Build history of the part. All positions in model axes, mm. A direction names the side the tool comes from. Coordinates: 2 decimals unless noted, no trailing zeros. Loops run counter-clockwise (first coordinate to the right, second up) from the corner with the lowest first, then second, coordinate; pieces in that order, holes last.
Item 1: 3-axis set-ups, long thin cutter, end or side, ignore diameter. For faces 1 (the face through (-37.38, 2, 24)), 2 (the face through (-88, -18.624, 13)), 3 (the face through (-177.41, 10.276, 9.806)): which of +Z, -Z, +X, -X, +Y, -Y reach the whole face in a straight line?
Item 2: Flat gauge pins, fed straight in: pin 1 (5 mm diameter, centred on y = 29, z = 13, fed in from -X); pin 2 (6 mm diameter, centred on x = -127.5, z = 20, fed in from -Y); pin 3 (11 mm diameter, centred on x = -157, z = 13.5, fed in from -Y). Where does each tip first touch, or does it go through?
Item 3: Cut at A-A (x = -41). List the corners of the cut face in (y, z), and give its area (3 significant figures).
Item 4: Cut at C-C (y = -13). List the corners of the cut face in (x, z).
Item 5: Cut at D-D (y = 28). List the corners of the cut face in (x, z), and give its area (3 significant figures).
Item 6: Mould opens along X. For faces 4 (the face through (16.557, 4, 13)), 5 (the face through (-152, -4.802, 11)), 6 (the face through (-164.888, 6, 11)) say: released by +X, released by -X, zero draft, split by the parting line, or undercut.
Item 7: Drill centre lines: line 1 along X through (y, z) = (-3.5, 25); line 2 along X through (y, z) = (18, 15.5); line 3 along Y through (x, z) = (-120, 23). Where is each one in solid material? Low to high.
Item 8: Cut at B-B (y = -0.5). List the corners of the cut face in (x, z), and give its area (3 significant figures).
from build123d import *

# Parameters (mm, degrees)
F0_W      = 53.9365671575
F0_H      = 55.1624000072
F1_DEPTH  = 25.4
F2_W      = 18.6239220202
F2_H      = 16.7940715328
F2_W_2    = 25.7758889347
F3_DEPTH  = 102.108
F4_W      = 102.108
F4_H      = 13.8221322559
F4_H_2    = 17.5757771358
F5_DEPTH  = 4.318
F6_DEPTH  = 5.0270510837
F8_DEPTH  = 25.4
F9_R      = 2.6384462804
F10_DEPTH = 25.4
F11_R     = 2.54
F12_R     = 2.54


with BuildPart() as f1:
    # F0 (on Top) → F1 (new body)
    with BuildSketch(Plane.XY):
        with Locations((-10.4117374867, 4.1782557964)):
            Rectangle(F0_W, F0_H)
    extrude(amount=F1_DEPTH)

    # F2 (on face) → F3 (join)
    with BuildSketch(Plane(origin=(-37.3800210655, 0, 0), x_dir=(0, -1, 0), z_dir=(-1, 0, 0))):
        with Locations((9.3119610101, 13.4240868501)):
            Rectangle(F2_W, F2_H)
        with Locations((-12.8879444674, 13.4240868501)):
            Rectangle(F2_W_2, F2_H)
    extrude(amount=F3_DEPTH)

    # F4 (on face) → F5 (join)
    with BuildSketch(Plane.XY.offset(21.8211226165)):
        with Locations((-88.4340210655, -11.7128558923)):
            Rectangle(F4_W, F4_H)
        with Locations((-88.4340210655, 16.9880003668)):
            Rectangle(F4_W, F4_H_2)
    extrude(amount=F5_DEPTH)

    # F6 (add, through all): a face of the model
    f6_faces = [f1.faces().sort_by_distance(p)[0] for p in [
        (-88.4340210655, 3.5759834573, 5.0270510837),
    ]]
    extrude(f6_faces, amount=F6_DEPTH)

    # F7 (on face) → F8 (join)
    with BuildSketch(Plane(origin=(-139.4880210655, 0, 0), x_dir=(0, -1, 0), z_dir=(-1, 0, 0))):
        Polygon((-16.9880003668, 0), (4.8017897643, 0), (4.8017897643, 21.8211226165), (-8.2001117989, 21.8211226165), (-16.9880003668, 21.8211226165), align=None)
    extrude(amount=F8_DEPTH)

    # F9 (on face) → F10 (join)
    with BuildSketch(Plane(origin=(-164.8880210655, 0, 0), x_dir=(0, -1, 0), z_dir=(-1, 0, 0))):
        with Locations((-8.3315027878, 8.0225486308)):
            Circle(F9_R)
    extrude(amount=F10_DEPTH)

    # F11
    f11_edges = [f1.edges().sort_by_distance(p)[0] for p in [
        (-164.888021, 6.093105, 21.821123),
    ]]
    fillet(f11_edges, radius=F11_R)

    # F12
    f12_edges = [f1.edges().sort_by_distance(p)[0] for p in [
        (-164.888021, 6.093105, 0),
    ]]
    fillet(f12_edges, radius=F12_R)


solid = f1.part
Filled sheet:
1. face 1: +Z, -X
1. face 2: +Z, -Z, -X, -Y
1. face 3: -X
2. pin 1: stops at x = -37.38
2. pin 2: stops at y = -18.62
2. pin 3: stops at y = -4.8
3. outline: (-18.62, 0) - (25.78, 0) - (25.78, 26.14) - (8.2, 26.14) - (8.2, 21.82) - (-4.8, 21.82) - (-4.8, 26.14) - (-18.62, 26.14) - close
3. area: 1,100 mm2
4. outline: (-139.49, 0) - (16.56, 0) - (16.56, 25.4) - (-37.38, 25.4) - (-37.38, 26.14) - (-139.49, 26.14) - close
5. outline: (-37.38, 0) - (16.56, 0) - (16.56, 25.4) - (-37.38, 25.4) - close
5. area: 1,370 mm2
6. face 4: released by +X
6. face 5: zero draft
6. face 6: released by -X
7. line 1: x = -37.38 to 16.56
7. line 2: x = -139.49 to 16.56
7. line 3: y = -18.62 to -4.8, 8.2 to 25.78
8. outline: (-164.89, 2.54) arc R2.54 ccw to (-162.35, 0) - (16.56, 0) - (16.56, 25.4) - (-37.38, 25.4) - (-37.38, 21.82) - (-162.35, 21.82) arc R2.54 ccw to (-164.89, 19.28) - close
8. area: 4,150 mm2
